```python
from build123d import *

# Parameters (mm, degrees)
SKETCH1_R           = 1.65
SKETCH1_R_2         = 5
SKETCH1_W           = 30.68
SKETCH1_H           = 2.7
SKETCH1_W_2         = 12
BOSS_EXTRUDE1_DEPTH = 2.7


with BuildPart() as part:
    # Sketch1 → Boss-Extrude1 (new body)
    with BuildSketch(Plane(origin=(0, 0, 0), x_dir=(1, 0, 0), z_dir=(0, 1, 0))):
        with BuildLine():
            Line((-46, 0), (46, 0))
            ThreePointArc((46, 0), (62.780941571, 3.32568378), (77.025151087, 12.8))
            Line((77.025151087, 12.8), (46.015151087, 12.8))
            Line((46.015151087, 12.8), (46.015151087, 15.5))
            Line((46.015151087, 15.5), (73.995151087, 15.5))
            Line((73.995151087, 15.5), (73.995151087, 35.5))
            Line((73.995151087, 35.5), (30, 35.5))
            Line((30, 35.5), (30, 70.5))
            Line((30, 70.5), (30, 72.5))
            Line((30, 72.5), (-30, 72.5))
            Line((-30, 72.5), (-30, 70.5))
            Line((-30, 70.5), (-30, 35.5))
            Line((-30, 35.5), (-73.995151087, 35.5))
            Line((-73.995151087, 35.5), (-73.995151087, 15.5))
            Line((-73.995151087, 15.5), (-46.015151087, 15.5))
            Line((-46.015151087, 15.5), (-46.015151087, 12.8))
            Line((-46.015151087, 12.8), (-77.025151087, 12.8))
            ThreePointArc((-77.025151087, 12.8), (-62.780941571, 3.32568378), (-46, 0))
        make_face()
        with Locations((46, 28.5)):
            Circle(SKETCH1_R, mode=Mode.SUBTRACT)
        with Locations((46, 7)):
            Circle(SKETCH1_R, mode=Mode.SUBTRACT)
        with Locations((-46, 7)):
            Circle(SKETCH1_R, mode=Mode.SUBTRACT)
        with Locations((-46, 28.5)):
            Circle(SKETCH1_R, mode=Mode.SUBTRACT)
        with Locations((-27, 69.5)):
            Circle(SKETCH1_R, mode=Mode.SUBTRACT)
        with Locations((27, 69.5)):
            Circle(SKETCH1_R, mode=Mode.SUBTRACT)
        with Locations((0, 27)):
            Circle(SKETCH1_R_2, mode=Mode.SUBTRACT)
        with Locations((0, 14.15)):
            Rectangle(SKETCH1_W, SKETCH1_H, mode=Mode.SUBTRACT)
        with Locations((12, 46.85)):
            Rectangle(SKETCH1_W_2, SKETCH1_H, mode=Mode.SUBTRACT)
        with Locations((-12, 64.15)):
            Rectangle(SKETCH1_W_2, SKETCH1_H, mode=Mode.SUBTRACT)
        with Locations((12, 64.15)):
            Rectangle(SKETCH1_W_2, SKETCH1_H, mode=Mode.SUBTRACT)
        with Locations((-12, 46.85)):
            Rectangle(SKETCH1_W_2, SKETCH1_H, mode=Mode.SUBTRACT)
    extrude(amount=BOSS_EXTRUDE1_DEPTH)


solid = part.part
```
Model file for the job. Use its own axes, mm. A direction names the side the tool comes from. Give positions to 0.01 mm unless a question says otherwise; leave off trailing zeros. Loops run counter-clockwise (first coordinate to the right, second up) from the corner with the lowest first, then second, coordinate; pieces in that order, holes last. Notation, with made-up numbers: (-32.5, 36.25) - (-27.5, 36.25) arc R9 cw to (-27.5, 45.25) - close; hole circle Ø8 at (35.5, -13.75). An arc over 180 degrees is marked (long way). One line per item, written item: value. Start each with the question number.
1. Slice it at D-D (z = -28.5). List the corners of the cut face in (x, y), plus the area to 3 significant figures.
2. Probe L1, parallel to X at y = 0.25, z = -64.5; L2, parallel to Z at x = 8, y = 2.2; L3, parallel to X at y = 1.5, z = -69.5. List the from-to ranges inside material, lowest first. Write a range as from..to.
3. Slice it at C-C (y = 0.9). Give the number of separate pieces and of enclosed holes in the cut face, plus the area to 3 significant figures.
4. Which spindle directions (+Z, -Z, +X, -X, +Y, -Y) get a long thin tool onto all of the face, cutting with end or side? Do faces 5 (the flat face through (-73.995, 1, -26)), 6 (the flat face through (-12, 1, -48.2)), 7 (the flat face through (30, 1, -54)), 8 (the flat face through (-60, 1, -15.5)). Say none if no direction does.
5. Pin check, flat tips, straight feed: pin 1 (2.5 mm diameter, centred on x = 27, z = -69.5, fed in from -Y); pin 2 (1.3 mm diameter, centred on y = 2, z = -15, fed in from -X); pin 3 (1.4 mm diameter, centred on y = 1, z = -22.5, fed in from +X); pin 4 (1.3 mm diameter, centred on y = 0.5, z = -14.5, fed in from -X). Stop position of each tip, or through.
6. Pull direction X, two halves, no side cores. Call faces 1 (the flat face through (-30, 1, -54)), 2 (the flat face through (73.995, 1, -25)), 3 (the cylindrical face through (-1.08, 1.33, -22.12)), 4 (the flat face through (-1, 1, 0)): pulls with the +X half, pulls with the -X half, needs draft (parallel to the pull), parting line crosses it, or undercut.
7. Slice it at B-B (x = 65). List the corners of the cut face in (y, z), plus the area to 3 significant figures.
8. Slice it at A-A (z = -69.5). List the corners of the cut face in (x, y), plus the area to 3 significant figures.
Solution:
1. outline: (-74, 0) - (-47.65, 0) - (-47.65, 2.7) - (-74, 2.7) - close; (-44.35, 0) - (-4.77, 0) - (-4.77, 2.7) - (-44.35, 2.7) - close; (4.77, 0) - (44.35, 0) - (44.35, 2.7) - (4.77, 2.7) - close; (47.65, 0) - (74, 0) - (74, 2.7) - (47.65, 2.7) - close
1. area: 356 mm^2
2. L1: x = -30..-18, -6..6, 18..30
2. L2: z = -72.5..-65.5, -62.8..-48.2, -45.5..-15.5, -12.8..0
2. L3: x = -30..-28.65, -25.35..25.35, 28.65..30
3. separate pieces: 1
3. enclosed holes: 12
3. area: 6,810 mm^2
4. face 5: -Z, -X, +Y, -Y
4. face 6: +Y, -Y
4. face 7: -Z, +X, +Y, -Y
4. face 8: -X, +Y, -Y
5. pin 1: passes through
5. pin 2: stops at x = -74
5. pin 3: stops at x = 74
5. pin 4: stops at x = -46.02
6. face 1: pulls with the -X half
6. face 2: pulls with the +X half
6. face 3: undercut
6. face 4: needs draft
7. outline: (0, -35.5) - (2.7, -35.5) - (2.7, -15.5) - (0, -15.5) - close; (0, -12.8) - (2.7, -12.8) - (2.7, -4.31) - (0, -4.31) - close
7. area: 76.9 mm^2
8. outline: (-30, 0) - (-28.65, 0) - (-28.65, 2.7) - (-30, 2.7) - close; (-25.35, 0) - (25.35, 0) - (25.35, 2.7) - (-25.35, 2.7) - close; (28.65, 0) - (30, 0) - (30, 2.7) - (28.65, 2.7) - close
8. area: 144 mm^2
